Check sheet for the modelled part. Datum: model origin and axes. Units: mm. A direction names the side the tool comes from. Round coordinates to 2 decimals unless told otherwise and drop trailing zeros. Order: outer loops, then holes, each group sorted by start corner. A loop starts at its lowest first (then second) coordinate and runs counter-clockwise, first axis right, second up.
```python
from build123d import *

# Parameters (mm, degrees)
F0_W     = 4.8
F0_H     = 2
F0_W_2   = 2
F0_H_2   = 4.8
F1_DEPTH = 20
F2_R     = 4
F3_DEPTH = 50
F4_DEPTH = 6


with BuildPart() as f1:
    # F0 (on Front) → F1 (new body, symmetric)
    with BuildSketch(Plane.XZ):
        Polygon((10.3, -20), (10.3, -10.3), (2.4, -10.3), (-2.4, -10.3), (-10.3, -10.3), (-10.3, -2.4), (-10.3, 2.4), (-10.3, 10.3), (-2.4, 10.3), (2.4, 10.3), (10.3, 10.3), (10.3, 20), (-26, 20), (-26, -20), align=None)
        with Locations((0, -9.3)):
            Rectangle(F0_W, F0_H)
        with Locations((0, 9.3)):
            Rectangle(F0_W, F0_H)
        with Locations((-9.3, 0)):
            Rectangle(F0_W_2, F0_H_2)
    extrude(amount=F1_DEPTH, both=True)

    # F2 (on face) → F3 (cut)
    with BuildSketch(Plane.XY.offset(20)):
        with Locations((-18, 0)):
            Circle(F2_R)
    extrude(amount=-F3_DEPTH, mode=Mode.SUBTRACT)

    # F2 (on face) → F4 (cut)
    with BuildSketch(Plane.XY.offset(20)):
        Polygon((-11.5, -3.752777), (-11.5, 3.752777), (-18, 7.505553), (-24.5, 3.752777), (-24.5, -3.752777), (-18, -7.505553), align=None)
        with Locations((-18, 0)):
            Circle(F2_R, mode=Mode.SUBTRACT)
    extrude(amount=-F4_DEPTH, mode=Mode.SUBTRACT)


solid = f1.part
```
Item 1: Sectioned sample at A-A (z = 9). Record the cut outline in (x, y).
Answer:
outline: (-26, -20) - (-10.3, -20) - (-10.3, 20) - (-26, 20) - close; (-2.4, -20) - (2.4, -20) - (2.4, 20) - (-2.4, 20) - close; hole circle Ø8 at (-18, 0)
Item 2: Release check for a two-part mould opening along Z. For faces 5 (the flat face through (-14.7, 5.6, 17)), 6 (the flat face through (-15, -3, 14)), 7 (the flat face through (-9, 0, 2.4)) record: released by +Z, released by -Z, zero draft, split by the parting line, or undercut.
Answer:
face 5: zero draft
face 6: released by +Z
face 7: undercut
Item 3: Go/stop test with flat-tipped pins: P1, Ø4, axis at y = 4, z = -7, coming from the +X side; P2, Ø4, axis at y = 5.5, z = 5.5, coming from the +X side; P3, Ø1.4, axis at y = 8, z = 0.5, coming from the +X side. Record where each tip stops, or that it passes through.
Answer:
P1: stops at x = 2.4
P2: stops at x = -10.3
P3: stops at x = -8.3
Item 4: Sectioned sample at D-D (y = -9). Record the cut outline in (x, z), and give its area (3 significant figures).
Answer:
outline: (-26, -20) - (10.3, -20) - (10.3, -10.3) - (2.4, -10.3) - (2.4, -8.3) - (-2.4, -8.3) - (-2.4, -10.3) - (-10.3, -10.3) - (-10.3, -2.4) - (-8.3, -2.4) - (-8.3, 2.4) - (-10.3, 2.4) - (-10.3, 10.3) - (-2.4, 10.3) - (-2.4, 8.3) - (2.4, 8.3) - (2.4, 10.3) - (10.3, 10.3) - (10.3, 20) - (-26, 20) - close
area: 1,060 mm2
Item 5: Scan lines: line 1 along Z through (x, y) = (-9, -10); line 2 along Z through (x, y) = (6.5, 11.5); line 3 along Y through (x, z) = (-18, 0). Record each from-to range of solid material in increasing order.
Answer:
line 1: z = -20 to -10.3, -2.4 to 2.4, 10.3 to 20
line 2: z = -20 to -10.3, 10.3 to 20
line 3: y = -20 to -4, 4 to 20
Item 6: Sectioned sample at C-C (y = 0). Record the cut outline in (x, z), and give its area (3 significant figures).
Answer:
outline: (-26, -20) - (-22, -20) - (-22, 14) - (-24.5, 14) - (-24.5, 20) - (-26, 20) - close; (-14, -20) - (10.3, -20) - (10.3, -10.3) - (2.4, -10.3) - (2.4, -8.3) - (-2.4, -8.3) - (-2.4, -10.3) - (-10.3, -10.3) - (-10.3, -2.4) - (-8.3, -2.4) - (-8.3, 2.4) - (-10.3, 2.4) - (-10.3, 10.3) - (-2.4, 10.3) - (-2.4, 8.3) - (2.4, 8.3) - (2.4, 10.3) - (10.3, 10.3) - (10.3, 20) - (-11.5, 20) - (-11.5, 14) - (-14, 14) - close
area: 706 mm2
Item 7: Access from +Z, -Z, +X, -X, +Y, -Y to the whole of each face (thin tool, end or side, straight path). Record for faces 1 (the flat face through (-10.3, 0, -6)), 2 (the flat face through (-8, 0, 20)), 3 (the flat face through (2.4, 0, 9)), 4 (the flat face through (-14.8, -5.66, 17.04)).
Answer:
face 1: +Y, -Y
face 2: +Z, +X, -X, +Y, -Y
face 3: +X, +Y, -Y
face 4: +Z
Item 8: Sectioned sample at B-B (x = 6.5). Record the cut outline in (y, z).
Answer:
outline: (-20, -20) - (20, -20) - (20, -10.3) - (-20, -10.3) - close; (-20, 10.3) - (20, 10.3) - (20, 20) - (-20, 20) - close
